Read the model definition and answer for the solid it produces. Units are mm, in the model's axes. Round coordinates to 2 decimals unless told otherwise and drop trailing zeros. Write each loop counter-clockwise with the first axis right and the second up, starting at its lowest first coordinate (ties: lowest second). Pieces come first, ordered by that corner, then holes.
from build123d import *

# Parameters (mm, degrees)
F1_DEPTH = 6.35


with BuildPart() as f1:
    # F0 (on Top) → F1 (new body)
    with BuildSketch(Plane.XY):
        with BuildLine():
            ThreePointArc((-24.0592682489, 0), (-14.2371131165, 4.0684698676), (-10.1686432489, 13.890625))
            ThreePointArc((-10.1686432489, 13.890625), (-10.6419546741, 17.4857827611), (-12.0296335682, 20.8359365366))
            ThreePointArc((-12.0296335682, 20.8359365366), (-13.0777646274, 22.3968604248), (-14.3270898061, 23.8019400312))
            ThreePointArc((-14.3270898061, 23.8019400312), (-24.0592682489, 13.890625), (-27.7766296295, 0.5066537188))
            ThreePointArc((-27.7766296295, 0.5066537188), (-25.9351329578, 0.1272462548), (-24.0592682489, 0))
        make_face()
        with BuildLine():
            ThreePointArc((-14.3270898061, 23.8019400312), (-13.0777646274, 22.3968604248), (-12.0296335682, 20.8359365366))
            ThreePointArc((-12.0296335682, 20.8359365366), (-12.8573677792, 22.5241066045), (-13.4495398234, 24.30859375))
            ThreePointArc((-13.4495398234, 24.30859375), (-13.890625, 24.0592682489), (-14.3270898061, 23.8019400312))
        make_face()
        with BuildLine():
            ThreePointArc((-13.4495398234, 24.30859375), (-12.8573677792, 22.5241066045), (-12.0296335682, 20.8359365366))
            ThreePointArc((-12.0296335682, 20.8359365366), (1.0177e-06, 13.890625), (12.0296345859, 20.8359382993))
            ThreePointArc((12.0296345859, 20.8359382993), (12.8573681644, 22.5241075465), (13.4495398234, 24.30859375))
            ThreePointArc((13.4495398234, 24.30859375), (0, 27.78125), (-13.4495398234, 24.30859375))
        make_face()
        with BuildLine():
            ThreePointArc((-27.7766296295, -0.5066537188), (-25.9351329578, -0.1272462548), (-24.0592682489, 0))
            ThreePointArc((-24.0592682489, 0), (-25.9351329578, 0.1272462548), (-27.7766296295, 0.5066537188))
            ThreePointArc((-27.7766296295, 0.5066537188), (-27.78125, 0), (-27.7766296295, -0.5066537188))
        make_face()
        with BuildLine():
            ThreePointArc((-10.1686432489, -13.890625), (-14.2371131165, -4.0684698676), (-24.0592682489, 0))
            ThreePointArc((-24.0592682489, 0), (-25.9351329578, -0.1272462548), (-27.7766296295, -0.5066537188))
            ThreePointArc((-27.7766296295, -0.5066537188), (-24.0592682489, -13.890625), (-14.3270898061, -23.8019400312))
            ThreePointArc((-14.3270898061, -23.8019400312), (-13.0777652945, -22.3968612859), (-12.0296346574, -20.8359384232))
            ThreePointArc((-12.0296346574, -20.8359384232), (-10.641954956, -17.4857838132), (-10.1686432489, -13.890625))
        make_face()
        with BuildLine():
            ThreePointArc((-27.7766296295, 0.5066537188), (-24.0592682489, 13.890625), (-14.3270898061, 23.8019400312))
            ThreePointArc((-14.3270898061, 23.8019400312), (-36.0889023733, 20.8359375), (-27.7766296295, 0.5066537188))
        make_face()
        with BuildLine():
            ThreePointArc((13.890625, 27.78125), (-1.7502783753, 41.5611624997), (-13.4495398234, 24.30859375))
            ThreePointArc((-13.4495398234, 24.30859375), (0, 27.78125), (13.4495398234, 24.30859375))
            ThreePointArc((13.4495398234, 24.30859375), (13.7799124997, 26.0309716247), (13.890625, 27.78125))
        make_face()
        with BuildLine():
            ThreePointArc((13.4495398234, 24.30859375), (12.8573681644, 22.5241075465), (12.0296345859, 20.8359382993))
            ThreePointArc((12.0296345859, 20.8359382993), (13.0777652506, 22.3968612294), (14.3270898061, 23.8019400312))
            ThreePointArc((14.3270898061, 23.8019400312), (13.890625, 24.0592682489), (13.4495398234, 24.30859375))
        make_face()
        with BuildLine():
            ThreePointArc((14.3270898061, 23.8019400312), (13.0777652506, 22.3968612294), (12.0296345859, 20.8359382993))
            ThreePointArc((12.0296345859, 20.8359382993), (12.0296338937, 6.9453128996), (24.0592682489, 0))
            ThreePointArc((24.0592682489, 0), (25.9351329578, 0.1272462548), (27.7766296295, 0.5066537188))
            ThreePointArc((27.7766296295, 0.5066537188), (24.0592682489, 13.890625), (14.3270898061, 23.8019400312))
        make_face()
        with BuildLine():
            ThreePointArc((-14.3270898061, -23.8019400312), (-24.0592682489, -13.890625), (-27.7766296295, -0.5066537188))
            ThreePointArc((-27.7766296295, -0.5066537188), (-36.0889023733, -20.8359375), (-14.3270898061, -23.8019400312))
        make_face()
        with BuildLine():
            ThreePointArc((37.9498932489, 13.890625), (29.4334389621, 26.6995184743), (14.3270898061, 23.8019400312))
            ThreePointArc((14.3270898061, 23.8019400312), (24.0592682489, 13.890625), (27.7766296295, 0.5066537188))
            ThreePointArc((27.7766296295, 0.5066537188), (35.1178833479, 5.4848832135), (37.9498932489, 13.890625))
        make_face()
        with BuildLine():
            ThreePointArc((27.7766296295, 0.5066537188), (25.9351329578, 0.1272462548), (24.0592682489, 0))
            ThreePointArc((24.0592682489, 0), (25.9351329578, -0.1272462548), (27.7766296295, -0.5066537188))
            ThreePointArc((27.7766296295, -0.5066537188), (27.7800948833, -0.2533373929), (27.78125, 0))
            ThreePointArc((27.78125, 0), (27.7800948833, 0.2533373929), (27.7766296295, 0.5066537188))
        make_face()
        with BuildLine():
            ThreePointArc((27.7766296295, -0.5066537188), (25.9351329578, -0.1272462548), (24.0592682489, 0))
            ThreePointArc((24.0592682489, 0), (12.0296338267, -6.9453130157), (12.0296347199, -20.8359385313))
            ThreePointArc((12.0296347199, -20.8359385313), (13.0777653327, -22.3968613353), (14.3270898061, -23.8019400312))
            ThreePointArc((14.3270898061, -23.8019400312), (24.0592682489, -13.890625), (27.7766296295, -0.5066537188))
        make_face()
        with BuildLine():
            ThreePointArc((12.0296347199, -20.8359385313), (6.25e-08, -13.890625), (-12.0296346574, -20.8359384232))
            ThreePointArc((-12.0296346574, -20.8359384232), (-12.8573681914, -22.5241076127), (-13.4495398234, -24.30859375))
            ThreePointArc((-13.4495398234, -24.30859375), (0, -27.78125), (13.4495398234, -24.30859375))
            ThreePointArc((13.4495398234, -24.30859375), (12.8573682151, -22.5241076705), (12.0296347199, -20.8359385313))
        make_face()
        with BuildLine():
            ThreePointArc((-13.4495398234, -24.30859375), (-12.8573681914, -22.5241076127), (-12.0296346574, -20.8359384232))
            ThreePointArc((-12.0296346574, -20.8359384232), (-13.0777652945, -22.3968612859), (-14.3270898061, -23.8019400312))
            ThreePointArc((-14.3270898061, -23.8019400312), (-13.890625, -24.0592682489), (-13.4495398234, -24.30859375))
        make_face()
        with BuildLine():
            ThreePointArc((37.9498932489, -13.890625), (35.1178833479, -5.4848832135), (27.7766296295, -0.5066537188))
            ThreePointArc((27.7766296295, -0.5066537188), (24.0592682489, -13.890625), (14.3270898061, -23.8019400312))
            ThreePointArc((14.3270898061, -23.8019400312), (29.4334389621, -26.6995184743), (37.9498932489, -13.890625))
        make_face()
        with BuildLine():
            ThreePointArc((14.3270898061, -23.8019400312), (13.0777653327, -22.3968613353), (12.0296347199, -20.8359385313))
            ThreePointArc((12.0296347199, -20.8359385313), (12.8573682151, -22.5241076705), (13.4495398234, -24.30859375))
            ThreePointArc((13.4495398234, -24.30859375), (13.890625, -24.0592682489), (14.3270898061, -23.8019400312))
        make_face()
        with BuildLine():
            ThreePointArc((13.4495398234, -24.30859375), (0, -27.78125), (-13.4495398234, -24.30859375))
            ThreePointArc((-13.4495398234, -24.30859375), (-1.7502783753, -41.5611624997), (13.890625, -27.78125))
            ThreePointArc((13.890625, -27.78125), (13.7799124997, -26.0309716247), (13.4495398234, -24.30859375))
        make_face()
        with BuildLine():
            ThreePointArc((-12.0296335682, 20.8359365366), (-10.6419546741, 17.4857827611), (-10.1686432489, 13.890625))
            ThreePointArc((-10.1686432489, 13.890625), (-14.2371131165, 4.0684698676), (-24.0592682489, 0))
            ThreePointArc((-24.0592682489, 0), (-14.2371131165, -4.0684698676), (-10.1686432489, -13.890625))
            ThreePointArc((-10.1686432489, -13.890625), (-10.641954956, -17.4857838132), (-12.0296346574, -20.8359384232))
            ThreePointArc((-12.0296346574, -20.8359384232), (6.25e-08, -13.890625), (12.0296347199, -20.8359385313))
            ThreePointArc((12.0296347199, -20.8359385313), (12.0296338267, -6.9453130157), (24.0592682489, 0))
            ThreePointArc((24.0592682489, 0), (12.0296338937, 6.9453128996), (12.0296345859, 20.8359382993))
            ThreePointArc((12.0296345859, 20.8359382993), (1.0177e-06, 13.890625), (-12.0296335682, 20.8359365366))
        make_face()
    extrude(amount=F1_DEPTH)


solid = f1.part
Q1. Straight lines are drawn through the part: probe 1 along X at (y, z) = (14, 3.25); probe 2 along Y at (x, z) = (34, 2.75); probe 3 along Y at (x, z) = (-32, 5). For each, find the intervals that lie inside material, in ascending order.
Verdict:
probe 1: x = -37.95 to 37.95
probe 2: y = -23.59 to -4.19, 4.19 to 23.59
probe 3: y = -25.29 to -2.49, 2.49 to 25.29
Q2. Section C-C (y = -21) is taken. Determine the outline of the cut face in (x, z), then the cut area to 3 significant figures.
Verdict:
outline: (-35.99, 0) - (35.99, 0) - (35.99, 6.35) - (-35.99, 6.35) - close
area: 457 mm2
Q3. Section A-A (z = 1.25) is taken. Determine the outline of the cut face in (x, y), then the cut area to 3 significant figures.
Verdict:
outline: (-27.78, -0.51) arc R13.89 ccw (long way) to (-14.33, -23.8) arc R27.78 ccw to (-13.45, -24.31) arc R13.89 ccw (long way) to (13.45, -24.31) arc R27.78 ccw to (14.33, -23.8) arc R13.89 ccw (long way) to (27.78, -0.51) arc R27.78 ccw to (27.78, 0.51) arc R13.89 ccw (long way) to (14.33, 23.8) arc R27.78 ccw to (13.45, 24.31) arc R13.89 ccw (long way) to (-13.45, 24.31) arc R27.78 ccw to (-14.33, 23.8) arc R13.89 ccw (long way) to (-27.78, 0.51) arc R27.78 ccw to start
area: 4,440 mm2
Q4. Determine the mould class of faces 1 (the cylindrical face through (-35.91, 21.14, 3.13)), 2 (the cylindrical face through (-36.26, -20.53, 3.13)), 3 (the flat face through (-1, 1, 6.35)) for opening direction X: pulls with the +X half, pulls with the -X half, needs draft (parallel to the pull), parting line crosses it, or undercut.
Verdict:
face 1: undercut
face 2: undercut
face 3: needs draft
Q5. Flat-ended cylindrical pins translate along their axes: pin 1 Ø1 at (y, z) = (29.5, 2.5) entering from -X; pin 2 Ø1 at (y, z) = (-25, 1) entering from +X; pin 3 Ø3 at (y, z) = (6, 4) entering from +X. Find the tip coordinate at first contact, or state that the pin passes through.
Verdict:
pin 1: stops at x = -13.84
pin 2: stops at x = 33.03
pin 3: stops at x = 36.39
Q6. Section B-B (x = -6.5) is taken. Determine the outline of the cut face in (y, z).
Verdict:
outline: (-40.06, 0) - (40.06, 0) - (40.06, 6.35) - (-40.06, 6.35) - close
